Source: CAD feature listing. Evaluate the final solid. Frame: model axes, mm. Face numbers are marked on the shaded views. Round coordinates to 2 decimals unless told otherwise and drop trailing zeros. Order: outer loops, then holes, each group sorted by start corner. A loop starts at its lowest first (then second) coordinate and runs counter-clockwise, first axis right, second up. Notation, with made-up numbers: (25.5, 5) - (38.5, 5) arc R8 cw to (38.5, 16) - close; hole circle Ø5 at (-36.75, -4.5). An arc over 180 degrees is marked (long way). Return JSON: item names as keys, results as strings. Group by question number.
1) Mould query, pull axis X, two halves, no side actions, for the marked faces 1, 2 and 3. Classes: pulls with the +X half, pulls with the -X half, needs draft (parallel to the pull), parting line crosses it, or undercut.
2) Section A-A, the plane z = 5. Return loops of the section in (x, y).
3) Ray query, line 1 (X direction, y = -10.75, z = -9.5); line 2 (X direction, y = -6, z = 8); line 3 (Z direction, x = 0, y = -13). Return the intervals inside material, ascending. Write a range as from..to.
4) Section D-D, the plane z = 17.5. Return loops of the section in (x, y).
5) Contact query for flat-ended pins moving along their axis: P1, Ø8, axis at y = -4.5, z = -24, coming from the -X side; P2, Ø5, axis at x = 62, y = -13.5, coming from the -Z side; P3, Ø4, axis at y = -4.5, z = 21, coming from the -X side; P4, Ø22.5, axis at x = 115.2, z = 0, coming from the +Y side. Output: stop coordinate, or through.
6) Section C-C, the plane x = 103.5. Return loops of the section in (y, z), plus the area to 3 significant figures.
7) Section B-B, the plane y = -3. Return loops of the section in (x, z), plus the area to 3 significant figures.
```python
from build123d import *

# Parameters (mm, degrees)
F0_R     = 22.8532905428
F0_R_2   = 14.1278184646
F1_DEPTH = 25.4


with BuildPart() as f1:
    # F0 (on Front) → F1 (new body)
    with BuildSketch(Plane.XZ):
        with BuildLine():
            Line((6.9627707482, 36.2147105875), (0, 36.8779804142))
            ThreePointArc((0, 36.8779804142), (-36.8779804142, 0), (0, -36.8779804142))
            Line((0, -36.8779804142), (6.9627707482, -36.2147105875))
            ThreePointArc((6.9627707482, -36.2147105875), (28.4320098015, -23.4862993695), (36.8779804142, 0))
            ThreePointArc((36.8779804142, 0), (28.4320098015, 23.4862993695), (6.9627707482, 36.2147105875))
        make_face()
        Circle(F0_R, mode=Mode.SUBTRACT)
        with BuildLine():
            Line((117.6412233187, 25.6715402452), (6.9627707482, 36.2147105875))
            ThreePointArc((6.9627707482, 36.2147105875), (28.4320098015, 23.4862993695), (36.8779804142, 0))
            ThreePointArc((36.8779804142, 0), (28.4320098015, -23.4862993695), (6.9627707482, -36.2147105875))
            Line((6.9627707482, -36.2147105875), (117.6412233187, -25.6715402452))
            ThreePointArc((117.6412233187, -25.6715402452), (89.4080124161, 0), (117.6412233187, 25.6715402452))
        make_face()
        with BuildLine():
            ThreePointArc((140.9835197666, 0), (134.2754816057, 17.3485646526), (117.6412233187, 25.6715402452))
            ThreePointArc((117.6412233187, 25.6715402452), (89.4080124161, 0), (117.6412233187, -25.6715402452))
            ThreePointArc((117.6412233187, -25.6715402452), (134.2754816057, -17.3485646526), (140.9835197666, 0))
        make_face()
        with Locations((115.1957660913, 0)):
            Circle(F0_R_2, mode=Mode.SUBTRACT)
    extrude(amount=F1_DEPTH)


solid = f1.part
```
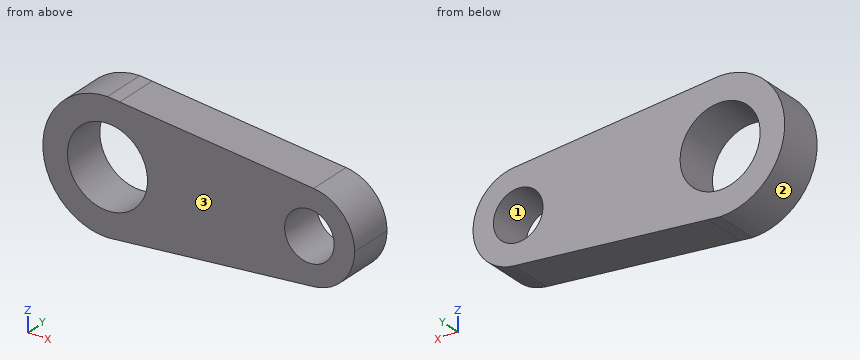
Geometry check:
{
 "1": {"face 1": "undercut", "face 2": "pulls with the -X half", "face 3": "needs draft"},
 "2": {"outline": "(-36.54, -25.4) - (-22.3, -25.4) - (-22.3, 0) - (-36.54, 0) - close; (22.3, -25.4) - (101.98, -25.4) - (101.98, 0) - (22.3, 0) - close; (128.41, -25.4) - (140.49, -25.4) - (140.49, 0) - (128.41, 0) - close"},
 "3": {"line 1": "-35.63..-20.79, 20.79..104.74, 125.65..139.17", "line 2": "-36..-21.41, 21.41..103.55, 126.84..139.71", "line 3": "-36.88..-22.85, 22.85..36.88"},
 "4": {"outline": "(-32.46, -25.4) - (-14.7, -25.4) - (-14.7, 0) - (-32.46, 0) - close; (14.7, -25.4) - (134.14, -25.4) - (134.14, 0) - (14.7, 0) - close"},
 "5": {"P1": "x = -30.98", "P2": "z = -31.21", "P3": "x = -31.61", "P4": "through"},
 "6": {"outline": "(-25.4, -27.02) - (0, -27.02) - (0, -7.92) - (-25.4, -7.92) - close; (-25.4, 7.92) - (0, 7.92) - (0, 27.02) - (-25.4, 27.02) - close", "area": "970 mm2"},
 "7": {"outline": "(0, -36.88) - (117.64, -25.67) arc R25.79 ccw to (117.64, 25.67) - (0, 36.88) arc R36.88 ccw to start; hole circle Ø45.71 at (0, 0); hole circle Ø28.26 at (115.2, 0)", "area": "8,150 mm2"}
}
